```python
from build123d import *

# Parameters (mm, degrees)
SKETCH1_R           = 15
SKETCH1_R_2         = 2
SKETCH1_W           = 20
SKETCH1_H           = 13
BOSS_EXTRUDE1_DEPTH = 5
CUT_EXTRUDE2_START  = -3
SKETCH6_R           = 3
SKETCH6_R_2         = 2
CUT_EXTRUDE2_DEPTH  = 3
FILLET1_R           = 1
SKETCH7_R           = 1.25
CUT_EXTRUDE3_DEPTH  = 15
SKETCH9_R           = 2
CUT_EXTRUDE4_DEPTH  = 8
SKETCH8_R           = 2
CUT_EXTRUDE5_DEPTH  = 8


with BuildPart() as part:
    # Sketch1 → Boss-Extrude1 (new body)
    with BuildSketch(Plane.XY):
        Polygon((0, 90), (0, 0), (400, 0), (400, 90), (340, 90), (340, 86), (292, 86), (292, 90), (108, 90), (108, 86), (60, 86), (60, 90), align=None)
        with Locations((123, 30)):
            Circle(SKETCH1_R, mode=Mode.SUBTRACT)
        with Locations((277, 30)):
            Circle(SKETCH1_R, mode=Mode.SUBTRACT)
        with Locations((2.5, 45)):
            Circle(SKETCH1_R_2, mode=Mode.SUBTRACT)
        with Locations((50, 53.5)):
            Rectangle(SKETCH1_W, SKETCH1_H, mode=Mode.SUBTRACT)
        with Locations((85, 53.5)):
            Rectangle(SKETCH1_W, SKETCH1_H, mode=Mode.SUBTRACT)
        with BuildLine():
            ThreePointArc((160, 50), (150, 60), (160, 70))
            Line((160, 70), (240, 70))
            ThreePointArc((240, 70), (250, 60), (240, 50))
            Line((240, 50), (160, 50))
        make_face(mode=Mode.SUBTRACT)
        with Locations((315, 53.5)):
            Rectangle(SKETCH1_W, SKETCH1_H, mode=Mode.SUBTRACT)
        with Locations((397.5, 45)):
            Circle(SKETCH1_R_2, mode=Mode.SUBTRACT)
        with Locations((350, 53.5)):
            Rectangle(SKETCH1_W, SKETCH1_H, mode=Mode.SUBTRACT)
    extrude(amount=BOSS_EXTRUDE1_DEPTH)

    # Sketch6 → Cut-Extrude2 (cut)
    # profile 1 of 2: a face of its own
    with BuildSketch(Plane.XY.offset(5).offset(CUT_EXTRUDE2_START)):
        with Locations((397.5, 45)):
            Circle(SKETCH6_R)
        with Locations((397.5, 45)):
            Circle(SKETCH6_R_2, mode=Mode.SUBTRACT)
    # profile 2 of 2: a face of its own
    with BuildSketch(Plane.XY.offset(5).offset(CUT_EXTRUDE2_START)):
        with Locations((2.5, 45)):
            Circle(SKETCH6_R)
        with Locations((2.5, 45)):
            Circle(SKETCH6_R_2, mode=Mode.SUBTRACT)
    extrude(amount=CUT_EXTRUDE2_DEPTH, mode=Mode.SUBTRACT)

    # Fillet1
    fillet1_edges = [part.edges().sort_by_distance(p)[0] for p in [
        (340, 60, 2.5),
        (340, 47, 2.5),
        (360, 47, 2.5),
        (360, 60, 2.5),
        (305, 60, 2.5),
        (305, 47, 2.5),
        (325, 47, 2.5),
        (325, 60, 2.5),
        (75, 60, 2.5),
        (75, 47, 2.5),
        (95, 47, 2.5),
        (95, 60, 2.5),
        (40, 60, 2.5),
        (40, 47, 2.5),
        (60, 47, 2.5),
        (60, 60, 2.5),
        (60, 86, 2.5),
        (108, 86, 2.5),
        (292, 86, 2.5),
        (340, 86, 2.5),
    ]]
    fillet(fillet1_edges, radius=FILLET1_R)

    # Sketch7 → Cut-Extrude3 (cut)
    with BuildSketch(Plane.XZ):
        with Locations(Location((360, 2.5, 0), (0, 0, 270))):
            Circle(SKETCH7_R)
        with Locations(Location((40, 2.5, 0), (0, 0, 270))):
            Circle(SKETCH7_R)
    extrude(amount=-CUT_EXTRUDE3_DEPTH, mode=Mode.SUBTRACT)

    # Sketch9 → Cut-Extrude4 (cut)
    with BuildSketch(Plane(origin=(0, 86, 0), x_dir=(1, 0, 0), z_dir=(0, 1, 0))):
        with Locations(Location((330, -2.5, 0), (0, 0, 270))):
            Circle(SKETCH9_R)
        with Locations(Location((316, -2.5, 0), (0, 0, 270))):
            Circle(SKETCH9_R)
        with Locations(Location((302, -2.5, 0), (0, 0, 270))):
            Circle(SKETCH9_R)
    extrude(amount=-CUT_EXTRUDE4_DEPTH, mode=Mode.SUBTRACT)

    # Sketch8 → Cut-Extrude5 (cut)
    with BuildSketch(Plane(origin=(0, 86, 0), x_dir=(1, 0, 0), z_dir=(0, 1, 0))):
        with Locations(Location((70, -2.5, 0), (0, 0, 180))):
            Circle(SKETCH8_R)
        with Locations(Location((84, -2.5, 0), (0, 0, 180))):
            Circle(SKETCH8_R)
        with Locations(Location((98, -2.5, 0), (0, 0, 180))):
            Circle(SKETCH8_R)
    extrude(amount=-CUT_EXTRUDE5_DEPTH, mode=Mode.SUBTRACT)


solid = part.part
```
Input: part model. Units: mm. Frame: model coordinates. A direction names the side the tool comes from. Give positions to 0.01 mm unless a question says otherwise; leave off trailing zeros. Order: outer loops, then holes, each group sorted by start corner. A loop starts at its lowest first (then second) coordinate and runs counter-clockwise, first axis right, second up. Notation, with made-up numbers: (-18, 61.25) -> (7, 61.25) arc R36 ccw to (7, 96.25) -> close; hole circle Ø9 at (5.25, -24.5). An arc over 180 degrees is marked (long way). Write each question's results on one line, items separated by ' | '. Start each with the question number.
Item 1: Cut plane A-A on x = 123. Return the cut outline in (y, z), then the cut area to 3 significant figures.
Item 2: Set-up query: faces 3 (the cylindrical face through (250, 60, 2)), 4 (the flat face through (197, 46, 0)). Return all of +Z, -Z, +X, -X, +Y, -Y with unobstructed straight access to the full face (end or side cutting, diameter ignored); none if empty.
Item 3: Mould query, pull axis X, two halves, no side actions, for faces 1 (the flat face through (197, 46, 5)), 2 (the cylindrical face through (291.307, 34.506, 2.465)). Classes: pulls with the +X half, pulls with the -X half, needs draft (parallel to the pull), parting line crosses it, or undercut.
Item 4: Line query: line 1 (Y direction, x = 181, z = 4.55); line 2 (Z direction, x = 360, y = 10); line 3 (Y direction, x = 316, z = 3.85). Output: solid intervals per line, ascending.
Item 5: Cut plane C-C on y = 25. Return the cut outline in (x, z), then the cut area to 3 significant figures.
Item 6: Cut plane B-B on x = 194. Return the cut outline in (y, z), then the cut area to 3 significant figures.
Item 7: Contact query for flat-ended pins moving along their axis: P1, Ø2.5, axis at x = 312.5, z = 2, coming from the +Y side; P2, Ø5, axis at x = 397.5, y = 45, coming from the +Z side. Output: stop coordinate, or through.
Established:
1) outline: (0, 0) -> (15, 0) -> (15, 5) -> (0, 5) -> close; (45, 0) -> (90, 0) -> (90, 5) -> (45, 5) -> close | area: 300 mm^2
2) face 3: +Z, -Z | face 4: -Z, +X, -X, +Y, -Y
3) face 1: needs draft | face 2: undercut
4) line 1: 0 to 50, 70 to 90 | line 2: 0 to 1.25, 3.75 to 5 | line 3: 0 to 47, 60 to 78
5) outline: (0, 0) -> (108.86, 0) -> (108.86, 5) -> (0, 5) -> close; (137.14, 0) -> (262.86, 0) -> (262.86, 5) -> (137.14, 5) -> close; (291.14, 0) -> (400, 0) -> (400, 5) -> (291.14, 5) -> close | area: 1,720 mm^2
6) outline: (0, 0) -> (50, 0) -> (50, 5) -> (0, 5) -> close; (70, 0) -> (90, 0) -> (90, 5) -> (70, 5) -> close | area: 350 mm^2
7) P1: y = 86 | P2: z = 2
